from build123d import *

# Parameters (mm, degrees)
F1_DEPTH = 158.26371
F2_R     = 2.5
F3_DEPTH = 5
F4_R     = 0.5
F6_DEPTH = 25.401


with BuildPart() as f1:
    # F0 (on Front) → F1 (new body)
    with BuildSketch(Plane.XZ):
        Polygon((0, 3), (0, 0), (25.4, 0), (25.4, 25.4), (0, 25.4), (0, 22.225), (22.4, 22.225), (22.4, 3), align=None)
    extrude(amount=F1_DEPTH)

    # F2 (on face) → F3 (cut)
    with BuildSketch(Plane.XY.offset(25.4)):
        with Locations((6, -14.6)):
            Circle(F2_R)
        with Locations((6, -143.66371)):
            Circle(F2_R)
        with Locations((6, -243.66371)):
            Circle(F2_R)
        with Locations((6, -343.66371)):
            Circle(F2_R)
        with Locations((6, -443.66371)):
            Circle(F2_R)
    extrude(amount=-F3_DEPTH, mode=Mode.SUBTRACT)

    # F4
    f4_edges = [f1.edges().sort_by_distance(p)[0] for p in [
        (0, -79.131855, 25.4),
        (0, -79.131855, 22.225),
        (25.4, -79.131855, 25.4),
        (22.4, -79.131855, 3),
        (0, -79.131855, 3),
        (0, -79.131855, 0),
        (22.4, -79.131855, 22.225),
        (25.4, -79.131855, 0),
    ]]
    fillet(f4_edges, radius=F4_R)

    # F5 (on face) → F6 (cut, through all)
    with BuildSketch(Plane(origin=(0, 0, 0), x_dir=(0, -1, 0), z_dir=(-1, 0, 0))):
        Polygon((0, 25.4), (0, 22.225), (3.175, 25.4), align=None)
        Polygon((155.08871, 25.4), (158.26371, 22.225), (158.26371, 25.4), align=None)
    extrude(amount=-F6_DEPTH, mode=Mode.SUBTRACT)


solid = f1.part
Build history of the part. All positions in model axes, mm. A direction names the side the tool comes from. Coordinates: 2 decimals unless noted, no trailing zeros. Order: outer loops, then holes, each group sorted by start corner. A loop starts at its lowest first (then second) coordinate and runs counter-clockwise, first axis right, second up. Notation, with made-up numbers: M 72.25,9.5 L 79.25,9.5 A32 ccw 79.25,37.5 Z; hole C 25,73 d2. An arc over 180 degrees is marked long. One line per question, with ' | ' between items. Start each with the question number.
Q1. Saw through at C-C (y = -43.5). List the corners of the cut face in (x, z) (3 decimals).
Q2. Saw through at B-B (x = 6). List the corners of the cut face in (y, z) (3 decimals), then the cut area to 3 significant figures.
Q3. Saw through at D-D (z = 11.25). List the corners of the cut face in (x, y), then the cut area to 3 significant figures.
Q4. Saw through at A-A (y = -14.6). List the corners of the cut face in (x, z) (3 decimals), then the cut area to 3 significant figures.
Q5. Flat gauge pin, fed straight in: pin 1 Ø5.5 at (y, z) = (-89, 14) entering from -X. Where does the tip first touch, or does it go through?
Q6. Probe L1, parallel to Z at x = 2.25, y = -131.5 (3 decimals); L2, parallel to X at y = -146, z = 7; L3, parallel to Y at x = 6, z = 24.5 (3 decimals). List the from-to ranges inside material, lowest first. Write a range as from..to.
Q7. 3-axis set-ups, long thin cutter, end or side, ignore diameter. For faces 1 (the face through (11, -78, 22.225)), 2 (the face through (12.522, -156.654, 23.835)), 3 (the face through (7.15, -16.82, 23.83)): which of +Z, -Z, +X, -X, +Y, -Y reach the whole face in a straight line?
Q8. Two-plate mould, pull along Z, no slides. Class faces 4 (the face through (25.4, -78, 13)), 5 (the face through (11, -78, 3)), 6 (the face through (13, -78, 25.4)): +Z half, -Z half, draft (parallel to the pull), parting line (faces both ways), or undercut.
Check values:
1) outline: M 0,0.5 A0.5 ccw 0.5,0 L 24.9,0 A0.5 ccw 25.4,0.5 L 25.4,24.9 A0.5 ccw 24.9,25.4 L 0.5,25.4 A0.5 ccw 0,24.9 L 0,22.725 A0.5 ccw 0.5,22.225 L 21.9,22.225 A0.5 cw 22.4,21.725 L 22.4,3.5 A0.5 cw 21.9,3 L 0.5,3 A0.5 ccw 0,2.5 Z
2) outline: M -158.264,0 L 0,0 L 0,3 L -158.264,3 Z; M -158.264,22.225 L -146.164,22.225 L -146.164,25.4 L -155.089,25.4 Z; M -141.164,22.225 L -17.1,22.225 L -17.1,25.4 L -141.164,25.4 Z; M -12.1,22.225 L 0,22.225 L -3.175,25.4 L -12.1,25.4 Z | area: 935 mm2
3) outline: M 22.4,-158.26 L 25.4,-158.26 L 25.4,0 L 22.4,0 Z | area: 475 mm2
4) outline: M 0,0.5 A0.5 ccw 0.5,0 L 24.9,0 A0.5 ccw 25.4,0.5 L 25.4,24.9 A0.5 ccw 24.9,25.4 L 8.5,25.4 L 8.5,22.225 L 21.9,22.225 A0.5 cw 22.4,21.725 L 22.4,3.5 A0.5 cw 21.9,3 L 0.5,3 A0.5 ccw 0,2.5 Z; M 0,22.725 A0.5 ccw 0.5,22.225 L 3.5,22.225 L 3.5,25.4 L 0.5,25.4 A0.5 ccw 0,24.9 Z | area: 198 mm2
5) pin 1: stops at x = 22.4
6) L1: z = 0..3, 22.225..25.4 | L2: x = 22.4..25.4 | L3: y = -155.989..-146.164, -141.164..-17.1, -12.1..-2.275
7) face 1: -X, +Y, -Y | face 2: +Z, +X, -X, -Y | face 3: +Z
8) face 4: draft | face 5: undercut | face 6: +Z half
